The figure shows three views and two pictorial views of one solid part (mm, origin at its lowest corner). Answer the questions. Give positions to 0.01 mm unless a question says otherwise; leave off trailing zeros. Order: outer loops, then holes, each group sorted by start corner. A loop starts at its lowest first (then second) coordinate and runs counter-clockwise, first axis right, second up. Notation, with made-up numbers: (5.25, 20) -> (19.25, 20) arc R30 cw to (19.25, 46) -> close; hole circle Ø7 at (31, 58). An arc over 180 degrees is marked (long way). One line per item, written item: value. Start each with the question number.
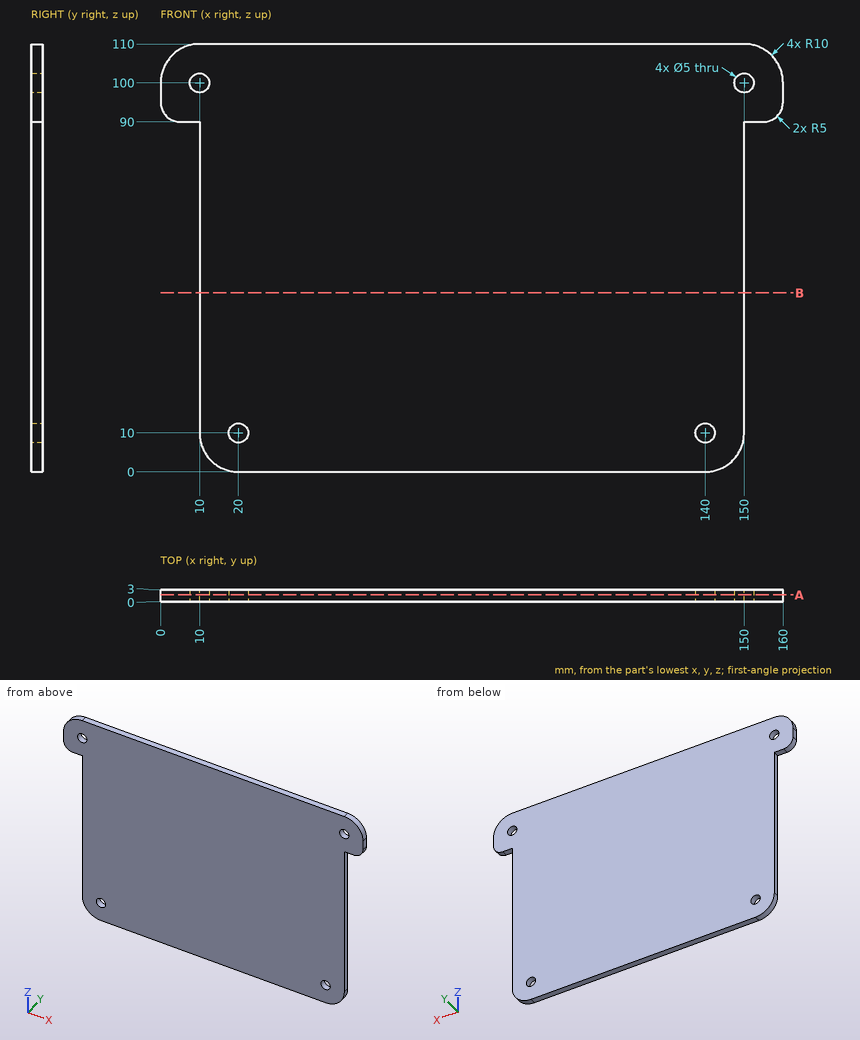
Item 1: Find the intervals of material crossed by line 1 (X direction, y = 1.6, z = 100); line 2 (X direction, y = 0.85, z = 10); line 3 (X direction, y = 0.4, z = 18), in increasing order. Write a range as from..to.
Item 2: A flat-ended cylindrical pin translates along its axis: pin 1 (1.5 mm diameter, centred on x = 151.5, y = 2, fed in from -Z). Find the tip coordinate at first contact, or state that the pin passes through.
Item 3: Find section B-B on z = 46. Write down the section's boundary in (x, y), then the cut area to 3 significant figures.
Item 4: Find section A-A on y = 1.7. Write down the section's boundary in (x, z), then the cut area to 3 significant figures.
Checks:
1. line 1: 0..7.5, 12.5..147.5, 152.5..160
1. line 2: 10..17.5, 22.5..137.5, 142.5..150
1. line 3: 10..150
2. pin 1: z = 90
3. outline: (10, 0) -> (150, 0) -> (150, 3) -> (10, 3) -> close
3. area: 420 mm2
4. outline: (0, 95) arc R5 ccw to (5, 90) -> (10, 90) -> (10, 10) arc R10 ccw to (20, 0) -> (140, 0) arc R10 ccw to (150, 10) -> (150, 90) -> (155, 90) arc R5 ccw to (160, 95) -> (160, 100) arc R10 ccw to (150, 110) -> (10, 110) arc R10 ccw to (0, 100) -> close; hole circle Ø5 at (10, 100); hole circle Ø5 at (20, 10); hole circle Ø5 at (140, 10); hole circle Ø5 at (150, 100)
4. area: 15,600 mm2
